Input: dimensioned drawing with shaded views. Units: mm. Origin: part minimum x, y, z. A direction names the side the tool comes from. Coordinates: 2 decimals unless noted, no trailing zeros. Order: outer loops, then holes, each group sorted by start corner. A loop starts at its lowest first (then second) coordinate and runs counter-clockwise, first axis right, second up. Notation, with made-up numbers: (71.5, 48.25) -> (96.5, 48.25) arc R19 cw to (96.5, 68.25) -> close; hole circle Ø9 at (-1, -25). An arc over 180 degrees is marked (long way). Answer as CSV lines item,"result".
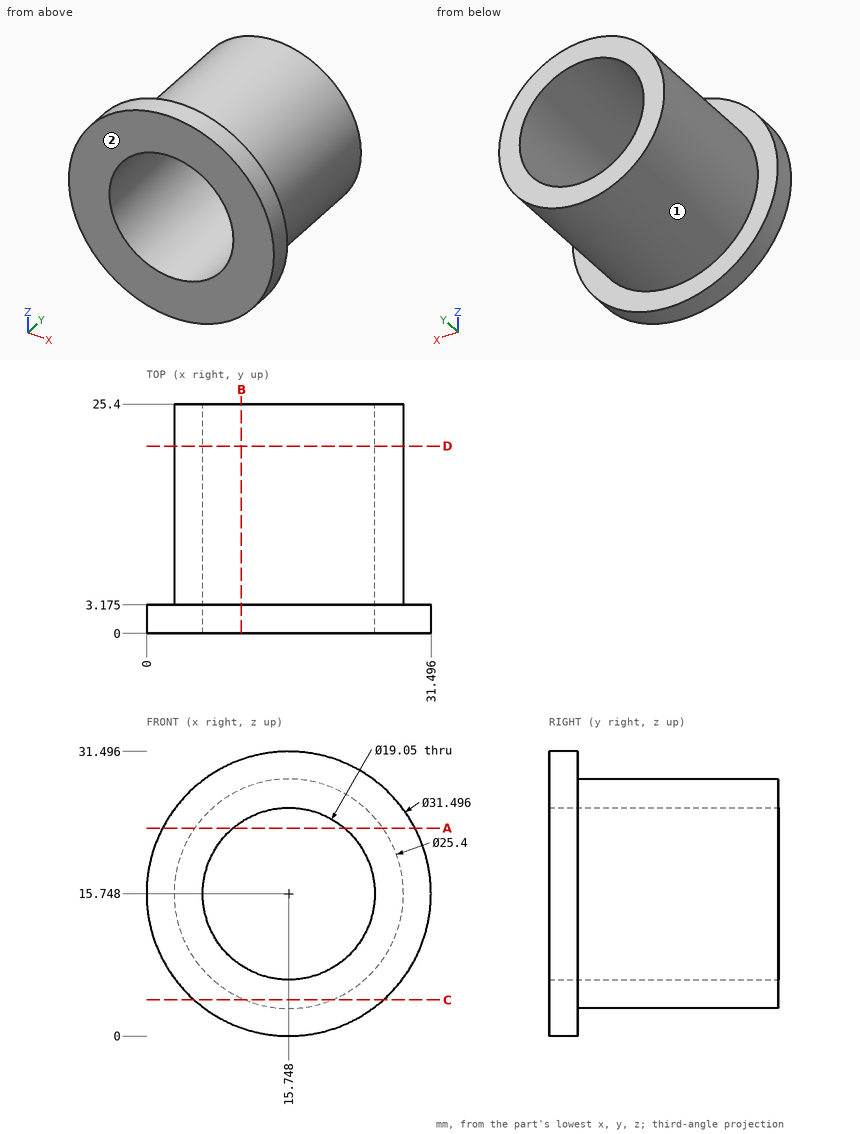
1. Cut plane C-C (z = 4). Return the cut outline in (x, y) (3 decimals), plus the area to 3 significant figures.
Findings:
outline,"(5.261, 0) -> (26.235, 0) -> (26.235, 3.175) -> (20.572, 3.175) -> (20.572, 25.4) -> (10.924, 25.4) -> (10.924, 3.175) -> (5.261, 3.175) -> close"
area,"281 mm2"
2. Cut plane B-B (x = 10.5). Return the cut outline in (y, z) (3 decimals), plus the area to 3 significant figures.
Findings:
outline,"(0, 0.9) -> (3.175, 0.9) -> (3.175, 4.183) -> (25.4, 4.183) -> (25.4, 7.799) -> (0, 7.799) -> close; (0, 23.697) -> (25.4, 23.697) -> (25.4, 27.313) -> (3.175, 27.313) -> (3.175, 30.596) -> (0, 30.596) -> close"
area,"205 mm2"
3. Cut plane D-D (y = 20.75). Return the cut outline in (x, z) (3 decimals), plus the area to 3 significant figures.
Findings:
outline,"circle Ø25.4 at (15.748, 15.748); hole circle Ø19.05 at (15.748, 15.748)"
area,"222 mm2"
4. Ray query, line 1 along X through (y, z) = (5.75, 16); line 2 along Y through (x, z) = (7, 6) (3 decimals); line 3 along X through (y, z) = (16, 19). Return the intervals inside material, ascending.
Findings:
line 1,"x = 3.05 to 6.23, 25.27 to 28.45"
line 2,"y = 0 to 3.175"
line 3,"x = 3.47 to 6.8, 24.7 to 28.02"
5. Reachability of the marked faces 1 and 2 from +Z, -Z, +X, -X, +Y, -Y: full face, straight path, thin tool, end or side. Return the list, or none.
Findings:
face 1,"+Y"
face 2,"+Z, -Z, +X, -X, -Y"
6. Cut plane A-A (z = 23). Return the cut outline in (x, y) (3 decimals).
Findings:
outline,"(1.769, 0) -> (9.573, 0) -> (9.573, 25.4) -> (5.322, 25.4) -> (5.322, 3.175) -> (1.769, 3.175) -> close; (21.923, 0) -> (29.727, 0) -> (29.727, 3.175) -> (26.174, 3.175) -> (26.174, 25.4) -> (21.923, 25.4) -> close"
7. Contact query for flat-ended pins moving along their axis: pin 1 (12 mm diameter, centred on x = 3.5, y = 3.5, fed in from -Z); pin 2 (1.5 mm diameter, centred on x = 4, y = 6, fed in from -Z); pin 3 (6 mm diameter, centred on x = 12.5, y = 4, fed in from -Z). Output: stop coordinate, or through.
Findings:
pin 1,"stops at z = 1.3"
pin 2,"stops at z = 9.4"
pin 3,"stops at z = 0"
